Build history of the part. All positions in model axes, mm. A direction names the side the tool comes from. Round coordinates to 2 decimals unless told otherwise and drop trailing zeros. Write each loop counter-clockwise with the first axis right and the second up, starting at its lowest first coordinate (ties: lowest second). Pieces come first, ordered by that corner, then holes. Notation, with made-up numbers: (35.5, 48) -> (74.5, 48) arc R21 cw to (74.5, 73) -> close; hole circle Ø10 at (83, 6.5). An arc over 180 degrees is marked (long way). One line per question, with ' | ' between items.
from build123d import *

# Parameters (mm, degrees)
F0_R     = 0.9
F1_DEPTH = 4
F2_R     = 0.9
F3_DEPTH = 1.2
F5_DEPTH = 0.2


with BuildPart() as f1:
    # F0 (on Right) → F1 (new body)
    with BuildSketch(Plane.YZ):
        with BuildLine():
            Line((20, 0), (0, 0))
            Line((0, 0), (0, -10))
            Line((0, -10), (15, -10))
            ThreePointArc((15, -10), (18.535534, -8.535534), (20, -5))
            Line((20, -5), (20, 0))
        make_face()
        with Locations((5, -5)):
            Circle(F0_R, mode=Mode.SUBTRACT)
        with Locations((15, -5)):
            Circle(F0_R, mode=Mode.SUBTRACT)
    extrude(amount=F1_DEPTH)

    # F2 (on face) → F3 (join)
    with BuildSketch(Plane.YZ.offset(4)):
        with BuildLine():
            Line((15, -3.1), (5, -3.1))
            ThreePointArc((5, -3.1), (3.1, -5), (5, -6.9))
            Line((5, -6.9), (15, -6.9))
            ThreePointArc((15, -6.9), (16.9, -5), (15, -3.1))
        make_face()
        with Locations((5, -5)):
            Circle(F2_R, mode=Mode.SUBTRACT)
        with Locations((15, -5)):
            Circle(F2_R, mode=Mode.SUBTRACT)
    extrude(amount=F3_DEPTH)

    # F4 (on face) → F5 (join)
    with BuildSketch(Plane(origin=(0, 0, 0), x_dir=(0, -1, 0), z_dir=(-1, 0, 0))):
        with BuildLine():
            ThreePointArc((-20, 2), (-21.414214, 1.414214), (-22, 0))
            Line((-22, 0), (-22, -5))
            ThreePointArc((-22, -5), (-19.949747, -9.949747), (-15, -12))
            Line((-15, -12), (0, -12))
            ThreePointArc((0, -12), (1.414214, -11.414214), (2, -10))
            Line((2, -10), (2, 0))
            ThreePointArc((2, 0), (1.414214, 1.414214), (0, 2))
            Line((0, 2), (-20, 2))
        make_face()
        with BuildLine():
            Line((-20, -5), (-20, 0))
            Line((-20, 0), (0, 0))
            Line((0, 0), (0, -10))
            Line((0, -10), (-15, -10))
            ThreePointArc((-15, -10), (-18.535534, -8.535534), (-20, -5))
        make_face(mode=Mode.SUBTRACT)
    extrude(amount=-F5_DEPTH)


solid = f1.part
(1) 3-axis set-ups, long thin cutter, end or side, ignore diameter. For faces 1 (the cylindrical face through (2, 18, -9)), 2 (the flat face through (2, 7, -10)), 3 (the cylindrical face through (4.6, 3.1, -5)), 4 (the cylindrical face through (4.6, 16.9, -5)): which of +Z, -Z, +X, -X, +Y, -Y reach the whole face in a straight line?
Calculated:
face 1: -Z, +X, +Y | face 2: -Z, +X, +Y, -Y | face 3: +X, -Y | face 4: +X, +Y
(2) Slice it at A-A (x = 2.8). Write the cut outline in (y, z).
Calculated:
outline: (0, -10) -> (15, -10) arc R5 ccw to (20, -5) -> (20, 0) -> (0, 0) -> close; hole circle Ø1.8 at (5, -5); hole circle Ø1.8 at (15, -5)
(3) Wall check: line 1 (Z direction, x = 3.6, y = 5); line 2 (X direction, y = 15.25, z = -9.25); line 3 (Y direction, x = 1.7, z = -3.5). Give the ranges that are in metal, low to high. Write a range as from..to.
Calculated:
line 1: -10..-5.9, -4.1..0 | line 2: 0..4 | line 3: 0..20
(4) Slice it at D-D (z = -9.25). Write the cut outline in (x, y).
Calculated:
outline: (0, -2) -> (0.2, -2) -> (0.2, 0) -> (4, 0) -> (4, 17.63) -> (0.2, 17.63) -> (0.2, 20.56) -> (0, 20.56) -> close
(5) Mould opens along Z. For faces 5 (the flat face through (5, 10, -6.9)), 6 (the cylindrical face through (2.564, 15.831, -5.345)), 7 (the cylindrical face through (2.564, 4.805, -5.879)), 8 (the flat face through (2, 10, 0)) say: pulls with the +Z half, pulls with the -Z half, needs draft (parallel to the pull), parting line crosses it, or undercut.
Calculated:
face 5: pulls with the -Z half | face 6: undercut | face 7: undercut | face 8: pulls with the +Z half
(6) Slice it at B-B (z = -1.25). Write the cut outline in (x, y), then the cut area to 3 significant figures.
Calculated:
outline: (0, -2) -> (0.2, -2) -> (0.2, 0) -> (4, 0) -> (4, 20) -> (0.2, 20) -> (0.2, 22) -> (0, 22) -> close | area: 80.8 mm2
(7) Drop flat-ended pins along their axis: pin 1 (1.3 mm diameter, centred on x = 4.5, y = 11.5, fed in from +Z); pin 2 (1.1 mm diameter, centred on y = 5, z = -5, fed in from +X); pin 3 (1.9 mm diameter, centred on x = 2, z = -3, fed in from +Y); pin 4 (2 mm diameter, centred on x = 4.5, y = 8.5, fed in from -Z). Give the stop position or say it passes through.
Calculated:
pin 1: z = 0 | pin 2: through | pin 3: y = 20 | pin 4: z = -10
(8) Slice it at C-C (y = 10). Write the cut outline in (x, z), then the cut area to 3 significant figures.
Calculated:
outline: (0, -12) -> (0.2, -12) -> (0.2, -10) -> (4, -10) -> (4, -6.9) -> (5.2, -6.9) -> (5.2, -3.1) -> (4, -3.1) -> (4, 0) -> (0.2, 0) -> (0.2, 2) -> (0, 2) -> close | area: 45.4 mm2
